from build123d import *

# Parameters (mm, degrees)
F1_DEPTH = 10
F3_D     = 4.5
F5_D     = 3


with BuildPart() as f1:
    # F0 (on Front) → F1 (new body)
    with BuildSketch(Plane.XZ):
        with BuildLine():
            Line((-17.5, 0), (-8, 0))
            Line((-8, 0), (8, 0))
            Line((8, 0), (17.5, 0))
            Line((17.5, 0), (17.5, 4))
            Line((17.5, 4), (8, 4))
            Line((8, 4), (8, 20))
            Line((8, 20), (0.75, 20))
            Line((0.75, 20), (0.75, 14.030819))
            ThreePointArc((0.75, 14.030819), (0, 5.9), (-0.75, 14.030819))
            Line((-0.75, 14.030819), (-0.75, 20))
            Line((-0.75, 20), (-8, 20))
            Line((-8, 20), (-8, 4))
            Line((-8, 4), (-17.5, 4))
            Line((-17.5, 4), (-17.5, 0))
        make_face()
    extrude(amount=F1_DEPTH)

    # F3 (through all)
    with Locations(Plane.XY.offset(4)):
        with Locations((-12.5, -5), (12.5, -5)):
            Hole(F3_D / 2)

    # F5 (through all)
    with Locations(Plane(origin=(-8, 0, 0), x_dir=(0, -1, 0), z_dir=(-1, 0, 0))):
        with Locations((5, 17)):
            Hole(F5_D / 2)


solid = f1.part
Can you work these out from the model? Positions are in its coordinate system, mm. A direction names the side the tool comes from. Give positions to 0.01 mm unless a question says otherwise; leave off trailing zeros. Loops run counter-clockwise (first coordinate to the right, second up) from the corner with the lowest first, then second, coordinate; pieces in that order, holes last. Notation, with made-up numbers: (-5, 70.25) - (23, 70.25) arc R14 ccw to (23, 78.25) - close; hole circle Ø7 at (33, 37.5). An arc over 180 degrees is marked (long way). One line per item, written item: value.
(1) If we mould it in two halves opening along Z, with no side actions, what happens to faces 1 (the face through (4.43, -6.11, 18.01)), 2 (the face through (0.75, -3.8, 18.4)), 3 (the face through (0, -5, 0))? For each: released by +Z, released by -Z, zero draft, split by the parting line, or undercut.
Verdict:
face 1: undercut
face 2: zero draft
face 3: released by -Z
(2) If we section it at B-B, the plane x = -12.5: List the corners of the cut face in (y, z) for me.
Verdict:
outline: (-10, 0) - (-7.25, 0) - (-7.25, 4) - (-10, 4) - close; (-2.75, 0) - (0, 0) - (0, 4) - (-2.75, 4) - close
(3) I'm going to push flat-ended pins straight in: pin 1 (5 mm diameter, centred on x = -14, y = -3, fed in from +Z); pin 2 (5 mm diameter, centred on y = -4.5, z = 12, fed in from -X); pin 3 (1.8 mm diameter, centred on y = -4.5, z = 15.5, fed in from +X). Where does each tip first touch, or does it pass through?
Verdict:
pin 1: z = 4
pin 2: x = -8
pin 3: x = 8
(4) I need wall thicknesses on line 1 along Z through (x, y) = (3.75, -5); line 2 along Z through (x, y) = (3.25, -5); line 3 along X through (y, z) = (-6.75, 10). Which ranges of each line are inside material? Lowest first, please.
Verdict:
line 1: 0 to 8.34, 11.66 to 15.5, 18.5 to 20
line 2: 0 to 7.5, 12.5 to 15.5, 18.5 to 20
line 3: -8 to -4.1, 4.1 to 8
(5) If we section it at C-C, the plane y = -5: List the corners of the cut face in (x, z) for me, plus the area to 3 significant figures.
Verdict:
outline: (-17.5, 0) - (-14.75, 0) - (-14.75, 4) - (-17.5, 4) - close; (-10.25, 0) - (10.25, 0) - (10.25, 4) - (8, 4) - (8, 15.5) - (0.75, 15.5) - (0.75, 14.03) arc R4.1 cw (long way) to (-0.75, 14.03) - (-0.75, 15.5) - (-8, 15.5) - (-8, 4) - (-10.25, 4) - close; (-8, 18.5) - (-0.75, 18.5) - (-0.75, 20) - (-8, 20) - close; (0.75, 18.5) - (8, 18.5) - (8, 20) - (0.75, 20) - close; (14.75, 0) - (17.5, 0) - (17.5, 4) - (14.75, 4) - close
area: 255 mm^2
(6) If we section it at D-D, the plane z = 17: List the corners of the cut face in (x, y) for me.
Verdict:
outline: (-8, -10) - (-0.75, -10) - (-0.75, -6.5) - (-8, -6.5) - close; (-8, -3.5) - (-0.75, -3.5) - (-0.75, 0) - (-8, 0) - close; (0.75, -10) - (8, -10) - (8, -6.5) - (0.75, -6.5) - close; (0.75, -3.5) - (8, -3.5) - (8, 0) - (0.75, 0) - close
(7) On a 3-axis mill with a long thin cutter (end or side, diameter ignored), from which of +Z, -Z, +X, -X, +Y, -Y can I reach the whole of each face in a straight line? I mean faces 4 (the face through (-8, -5, 12)), 5 (the face through (-0.2, 0, 5.7)), 6 (the face through (8, -5, 12)), 7 (the face through (-0.75, -3.8, 18.3)), 8 (the face through (17.5, -5, 2)). Say none if no direction works.
Verdict:
face 4: +Z, -X, +Y, -Y
face 5: +Z, -Z, +X, -X, +Y
face 6: +Z, +X, +Y, -Y
face 7: +Z, +Y, -Y
face 8: +Z, -Z, +X, +Y, -Y
(8) If we section it at A-A, the plane z = 10: List the corners of the cut face in (x, y) for me.
Verdict:
outline: (-8, -10) - (-4.1, -10) - (-4.1, 0) - (-8, 0) - close; (4.1, -10) - (8, -10) - (8, 0) - (4.1, 0) - close
